Design review of the part shown in the three views and the two pictorial views. Dimensions are in mm from the part's minimum x, y and z. A direction names the side the tool comes from. Round coordinates to 2 decimals unless told otherwise and drop trailing zeros. Order: outer loops, then holes, each group sorted by start corner. A loop starts at its lowest first (then second) coordinate and runs counter-clockwise, first axis right, second up. Notation, with made-up numbers: M 53,23.25 L 112,23.25 A3 cw 112,28.25 Z; hole C 65,44.5 d10. An arc over 180 degrees is marked long. Use a Markdown table: item, result. Add a question column.
(1) The part is to be moulded in two halves that separate along Z. For the marked faces 3, 4 and 5, say which applies: released by +Z, released by -Z, zero draft, split by the parting line, or undercut.
(2) Take a section at D-D (z = 12). Write out the cut boundary in (x, y), then the cut area to 3 significant figures.
(3) To check wall thickness, follow probe 1 along Z at (x, y) = (48, 8.5) (1 decimal); probe 2 along Z at (x, y) = (25.5, 32) (1 decimal); probe 3 along X at (y, z) = (50, 59) (1 decimal). State the ranges of each line that lie inside material, in increasing order. Write a range as from..to.
(4) Machinability: for the marked faces 1 and 2, which of the approach directions +Z, -Z, +X, -X, +Y, -Y give a long, thin tool a straight path to every point of the face, cutting with its end or side? Answer none if there is none.
(5) Take a section at A-A (z = 77). Write out the cut boundary in (x, y), then the cut area to 3 significant figures.
(6) For pin 1 (12 mm diameter, centred on x = 17, y = 43, fed in from -Z); pin 2 (4 mm diameter, centred on y = 31, z = 79.5, fed in from +X), all flat-tipped, find the tip position at first contact; note any pin that passes through.
(7) Take a section at C-C (y = 15.5). Write out the cut boundary in (x, z).
(8) Take a section at B-B (x = 27). Write out the cut boundary in (y, z).
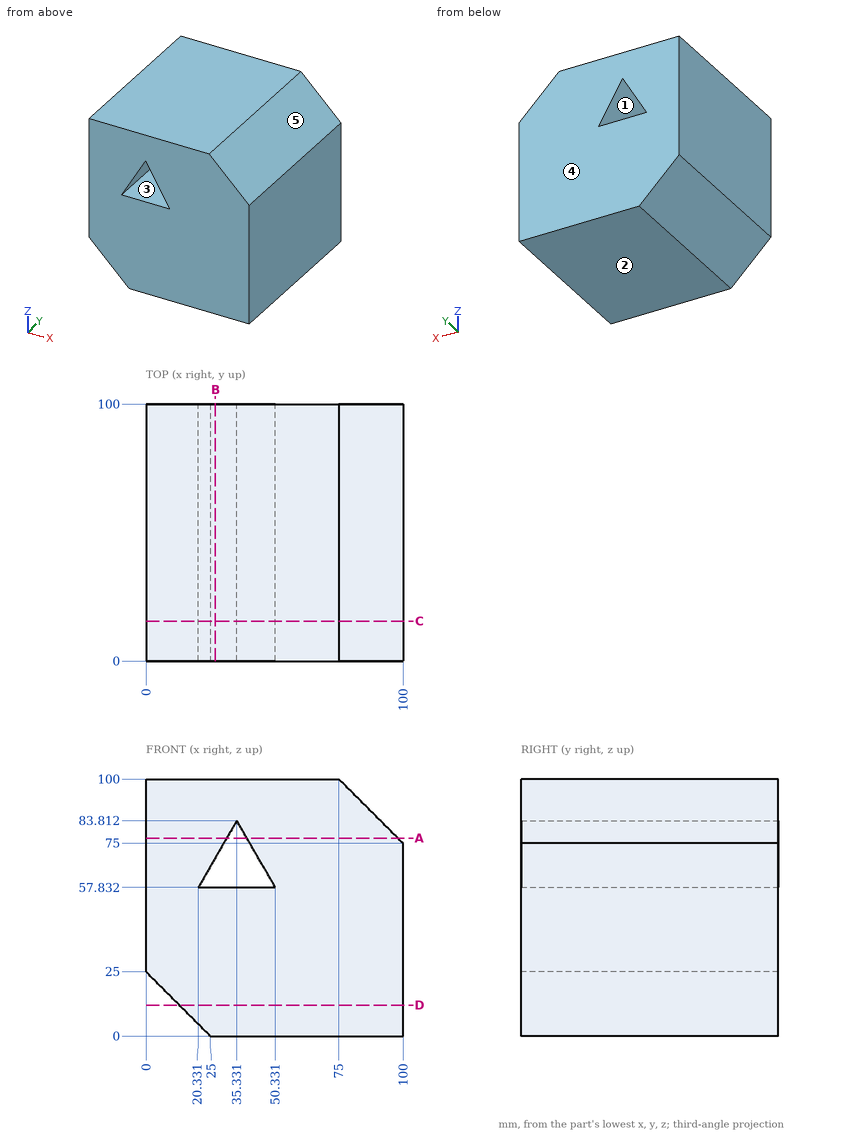
Verdict:
| question | item | result |
|---|---|---|
| 1 | face 3 | undercut |
| 1 | face 4 | zero draft |
| 1 | face 5 | released by +Z |
| 2 | outline | M 13,0 L 100,0 L 100,100 L 13,100 Z |
| 2 | area | 8,700 mm^2 |
| 3 | probe 1 | z = 0..57.8, 61.9..100 |
| 3 | probe 2 | z = 0..57.8, 66.8..100 |
| 3 | probe 3 | x = 0..21, 49.7..100 |
| 4 | face 1 | +Y, -Y |
| 4 | face 2 | -Z, +X, -X, +Y, -Y |
| 5 | outline | M 0,0 L 31.4,0 L 31.4,100 L 0,100 Z; M 39.26,0 L 98,0 L 98,100 L 39.26,100 Z |
| 5 | area | 9,010 mm^2 |
| 6 | pin 1 | stops at z = 2 |
| 6 | pin 2 | stops at x = 97.5 |
| 7 | outline | M 0,25 L 25,0 L 100,0 L 100,75 L 75,100 L 0,100 Z; hole M 20.33,57.83 L 50.33,57.83 L 35.33,83.81 Z |
| 8 | outline | M 0,0 L 100,0 L 100,57.83 L 0,57.83 Z; M 0,69.38 L 100,69.38 L 100,100 L 0,100 Z |
